from build123d import *

# Parameters (mm, degrees)
SKETCH2_W           = 150
SKETCH2_H           = 46
BOSS_EXTRUDE1_DEPTH = 6
CHAMFER2_SIZE       = 3
SKETCH3_R           = 2.5
CUT_EXTRUDE1_DEPTH  = 80.359939516
CHAMFER3_SIZE       = 1.5


with BuildPart() as part:
    # Sketch2 → Boss-Extrude1 (new, symmetric)
    with BuildSketch(Plane(origin=(0, 0, 0), x_dir=(1, 0, 0), z_dir=(0, 1, 0))):
        Rectangle(SKETCH2_W, SKETCH2_H)
    extrude(amount=BOSS_EXTRUDE1_DEPTH, both=True)

    # Chamfer2
    chamfer2_edges = [part.edges().sort_by_distance(p)[0] for p in [
        (-75, 6, 0),
        (0, 6, 23),
        (75, 6, 0),
        (0, 6, -23),
    ]]
    chamfer(chamfer2_edges, length=CHAMFER2_SIZE)

    # Sketch3 → Cut-Extrude1 (cut, through all)
    with BuildSketch(Plane(origin=(0, 6, 0), x_dir=(1, 0, 0), z_dir=(0, 1, 0))):
        with Locations(Location((-65, 8, 0), (0, 0, 270))):
            Circle(SKETCH3_R)
        with Locations(Location((-65, -7, 0), (0, 0, 270))):
            Circle(SKETCH3_R)
        with Locations(Location((65, 8, 0), (0, 0, 270))):
            Circle(SKETCH3_R)
        with Locations(Location((65, -7, 0), (0, 0, 270))):
            Circle(SKETCH3_R)
    extrude(amount=-CUT_EXTRUDE1_DEPTH, mode=Mode.SUBTRACT)

    # Chamfer3
    chamfer3_edges = [part.edges().sort_by_distance(p)[0] for p in [
        (-65, -6, 4.5),
        (65, -6, -10.5),
        (65, -6, 4.5),
        (-65, -6, -10.5),
    ]]
    chamfer(chamfer3_edges, length=CHAMFER3_SIZE)


solid = part.part
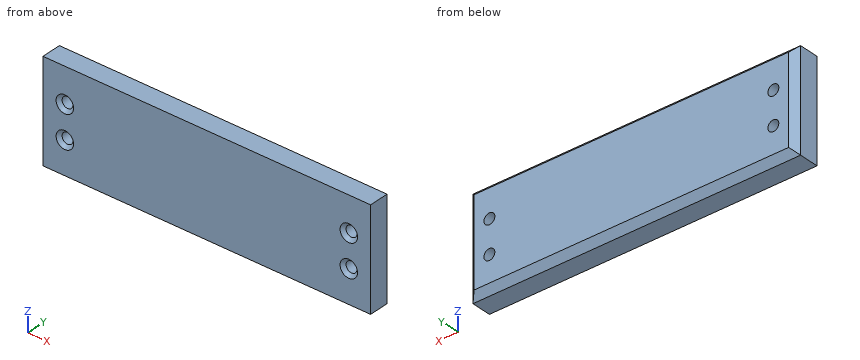
For this review, take the finished solid that the model builds, in its own axes (mm). Round coordinates to 2 decimals unless told otherwise and drop trailing zeros. Loops run counter-clockwise (first coordinate to the right, second up) from the corner with the lowest first, then second, coordinate; pieces in that order, holes last. Notation, with made-up numbers: (-20, 56.5) - (-10, 56.5) arc R27 ccw to (-10, 89.5) - close; hole circle Ø9 at (-32.5, 26). An arc over 180 degrees is marked (long way). One line per item, written item: value. Start each with the question number.
Item 1: Clearance check with flat-ended pins moving along their axes: pin 1 Ø6.5 at (x, z) = (65, -8) entering from -Y; pin 2 Ø6 at (x, z) = (-65, 7) entering from +Y; pin 3 Ø6 at (x, z) = (-65, -8) entering from -Y. State where each tip first meets the part, or that it passes through.
Item 2: Take a section at C-C (x = 4). Give the boundary of the cut face in (y, z).
Item 3: Take a section at B-B (z = 7). Give the boundary of the cut face in (x, y).
Item 4: For L1, parallel to X at y = 1.75, z = -8; L2, parallel to X at y = 4, z = 7; L3, parallel to Z at x = 0, y = 4.25, list the stretches that pass through material, from the lowest coordinate up.
Item 5: Take a section at A-A (x = 65). Give the boundary of the cut face in (y, z), plus the area to 4 significant figures.
Answer below:
1. pin 1: stops at y = -5.25
1. pin 2: stops at y = 6
1. pin 3: stops at y = -5
2. outline: (-6, -23) - (3, -23) - (6, -20) - (6, 20) - (3, 23) - (-6, 23) - close
3. outline: (-75, -6) - (-69, -6) - (-67.5, -4.5) - (-67.5, 6) - (-72, 6) - (-75, 3) - close; (-62.5, -4.5) - (-61, -6) - (61, -6) - (62.5, -4.5) - (62.5, 6) - (-62.5, 6) - close; (67.5, -4.5) - (69, -6) - (75, -6) - (75, 3) - (72, 6) - (67.5, 6) - close
4. L1: x = -75 to -67.5, -62.5 to 62.5, 67.5 to 75
4. L2: x = -74 to -67.5, -62.5 to 62.5, 67.5 to 74
4. L3: z = -21.75 to 21.75
5. outline: (-6, -23) - (3, -23) - (6, -20) - (6, -10.5) - (-4.5, -10.5) - (-6, -12) - close; (-6, -4) - (-4.5, -5.5) - (6, -5.5) - (6, 4.5) - (-4.5, 4.5) - (-6, 3) - close; (-6, 11) - (-4.5, 9.5) - (6, 9.5) - (6, 20) - (3, 23) - (-6, 23) - close
5. area: 418.5 mm2
